Work out the finished part from the listing and answer in its coordinate system (mm). Face numbers are marked on the shaded views. Coordinates: 2 decimals unless noted, no trailing zeros. Write each loop counter-clockwise with the first axis right and the second up, starting at its lowest first coordinate (ties: lowest second). Pieces come first, ordered by that corner, then holes. Notation, with made-up numbers: (57.5, 46.5) - (66.5, 46.5) arc R11 ccw to (66.5, 56.5) - close; hole circle Ø2 at (77, -37.5). An arc over 180 degrees is marked (long way). Use one line per item in the form item = value. Start each with the question number.
Item 1: A cutting plane is placed at B-B (z = -4). Write down the section's boundary in (x, y).
Item 2: A cutting plane is placed at C-C (x = -4). Write down the section's boundary in (y, z).
Item 3: A cutting plane is placed at A-A (y = 1.5). Give the number of separate pieces and of enclosed holes in the cut face, then the cut area to 3 significant figures.
Item 4: Determine the mould class of the marked faces 1 and 2 for opening direction X: released by +X, released by -X, zero draft, split by the parting line, or undercut.
Item 5: A cutting plane is placed at D-D (x = -103.5). Write down the section's boundary in (y, z), then the cut area to 3 significant figures.
Item 6: Consider probe 1 along X at (y, z) = (1.9, -4); probe 2 along X at (y, z) = (-0.4, -35.9); probe 3 along Z at (x, y) = (-4, -0.4). Determine where each line is inside the solid, lowest interval first.
Item 7: Given pin 1 (4 mm diameter, centred on x = -99, z = -10, fed in from -Y), flat-ended and moving along its own axis, determine where the tip first touches the part or whether it passes through.
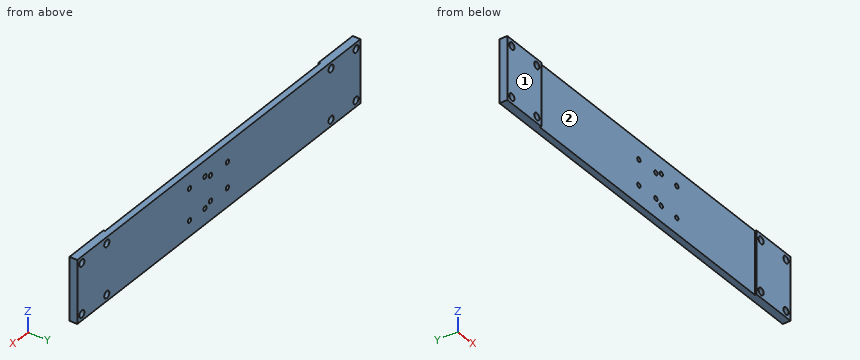
from build123d import *
from build123d.topology import SkipClean

# Parameters (mm, degrees)
SKETCH_1_W          = 250
SKETCH_1_H          = 39.9
EXTRUDE_1_DEPTH     = 4
SKETCH_2_R          = 1.45
CUT_EXTRUDE_1_DEPTH = 12
SKETCH_3_R          = 1.45
CUT_EXTRUDE_2_DEPTH = 12
SKETCH_7_R          = 2.25
CUT_EXTRUDE_6_DEPTH = 20
SKETCH_8_W          = 30
SKETCH_8_H          = 39.9
SKETCH_8_R          = 2.25
EXTRUDE_2_DEPTH     = 1


with BuildPart() as part:
    # Sketch 1 → Extrude 1 (new body)
    with BuildSketch(Plane(origin=(0, 0, 0), x_dir=(1, 0, 0), z_dir=(0, 1, 0))):
        with Locations((-125, 19.95)):
            Rectangle(SKETCH_1_W, SKETCH_1_H)
    extrude(amount=EXTRUDE_1_DEPTH)

    # Sketch 2 → Cut-Extrude 1 (cut)
    with BuildSketch(Plane(origin=(0, 4, 0), x_dir=(1, 0, 0), z_dir=(0, 1, 0))):
        with Locations(Location((-132.5, 27.95, 0), (0, 0, 270))):
            Circle(SKETCH_2_R)
        with Locations(Location((-117.5, 27.95, 0), (0, 0, 270))):
            Circle(SKETCH_2_R)
        with Locations(Location((-117.5, 11.95, 0), (0, 0, 270))):
            Circle(SKETCH_2_R)
        with Locations(Location((-132.5, 11.95, 0), (0, 0, 270))):
            Circle(SKETCH_2_R)
    extrude(amount=-CUT_EXTRUDE_1_DEPTH, mode=Mode.SUBTRACT)

    # Sketch 3 → Cut-Extrude 2 (cut)
    with BuildSketch(Plane(origin=(-275.091791604, 0, 105.376222054), x_dir=(-0.9999983055135633, 0, 0.0018409155336922224), z_dir=(0, -1, 0))):
        with Locations(Location((-162.553914397, 115.077169025, 0), (0, 0, 90.10547675))):
            Circle(SKETCH_3_R)
        with Locations(Location((-162.590548616, 134.977135305, 0), (0, 0, 90.10547675))):
            Circle(SKETCH_3_R)
        with Locations(Location((-176.303891098, 115.051856436, 0), (0, 0, 90.10547675))):
            Circle(SKETCH_3_R)
        with Locations(Location((-176.340525317, 134.951822716, 0), (0, 0, 90.10547675))):
            Circle(SKETCH_3_R)
    extrude(amount=-CUT_EXTRUDE_2_DEPTH, mode=Mode.SUBTRACT)

    # Sketch 7 → Cut-Extrude 6 (cut)
    with BuildSketch(Plane(origin=(0, 4, 0), x_dir=(1, 0, 0), z_dir=(0, 1, 0))):
        with Locations(Location((-246, 35.9, 0), (0, 0, 270))):
            Circle(SKETCH_7_R)
        with Locations(Location((-224, 35.9, 0), (0, 0, 270))):
            Circle(SKETCH_7_R)
        with Locations(Location((-224, 4, 0), (0, 0, 270))):
            Circle(SKETCH_7_R)
        with Locations(Location((-246, 4, 0), (0, 0, 270))):
            Circle(SKETCH_7_R)
        with Locations(Location((-4, 4, 0), (0, 0, 270))):
            Circle(SKETCH_7_R)
        with Locations(Location((-26, 4, 0), (0, 0, 270))):
            Circle(SKETCH_7_R)
        with Locations(Location((-26, 35.9, 0), (0, 0, 270))):
            Circle(SKETCH_7_R)
        with Locations(Location((-4, 35.9, 0), (0, 0, 270))):
            Circle(SKETCH_7_R)
    extrude(amount=-CUT_EXTRUDE_6_DEPTH, mode=Mode.SUBTRACT)

    # Sketch 8 → Extrude 2 (add)
    # profile 1 of 2: a face of its own
    with SkipClean():  # the faces are left unmerged after this step: merging them gives an invalid solid
        with BuildSketch(Plane.XZ):
            with Locations((-235, -19.95)):
                Rectangle(SKETCH_8_W, SKETCH_8_H)
            with Locations(Location((-224, -35.9, 0), (0, 0, 90))):
                Circle(SKETCH_8_R, mode=Mode.SUBTRACT)
            with Locations(Location((-246, -35.9, 0), (0, 0, 90))):
                Circle(SKETCH_8_R, mode=Mode.SUBTRACT)
            with Locations(Location((-224, -4, 0), (0, 0, 270))):
                Circle(SKETCH_8_R, mode=Mode.SUBTRACT)
            with Locations(Location((-246, -4, 0), (0, 0, 270))):
                Circle(SKETCH_8_R, mode=Mode.SUBTRACT)
        # profile 2 of 2: a face of its own
        with BuildSketch(Plane.XZ):
            with Locations((-15, -19.95)):
                Rectangle(SKETCH_8_W, SKETCH_8_H)
            with Locations(Location((-4, -35.9, 0), (0, 0, 270))):
                Circle(SKETCH_8_R, mode=Mode.SUBTRACT)
            with Locations(Location((-26, -35.9, 0), (0, 0, 270))):
                Circle(SKETCH_8_R, mode=Mode.SUBTRACT)
            with Locations(Location((-4, -4, 0), (0, 0, 90))):
                Circle(SKETCH_8_R, mode=Mode.SUBTRACT)
            with Locations(Location((-26, -4, 0), (0, 0, 90))):
                Circle(SKETCH_8_R, mode=Mode.SUBTRACT)
        extrude(amount=EXTRUDE_2_DEPTH)
    add(part.part.scale(1), mode=Mode.REPLACE)  # the faces are merged on a copy


solid = part.part
Answer:
q1.outline = (-250, -1) - (-248.25, -1) - (-248.25, 4) - (-250, 4) - close; (-243.75, -1) - (-226.25, -1) - (-226.25, 4) - (-243.75, 4) - close; (-221.75, -1) - (-220, -1) - (-220, 0) - (-30, 0) - (-30, -1) - (-28.25, -1) - (-28.25, 4) - (-221.75, 4) - close; (-23.75, -1) - (-6.25, -1) - (-6.25, 4) - (-23.75, 4) - close; (-1.75, -1) - (0, -1) - (0, 4) - (-1.75, 4) - close
q2.outline = (-1, -39.9) - (4, -39.9) - (4, -38.15) - (-1, -38.15) - close; (-1, -33.65) - (4, -33.65) - (4, -6.25) - (-1, -6.25) - close; (-1, -1.75) - (4, -1.75) - (4, 0) - (-1, 0) - close
q3.separate_pieces = 1
q3.enclosed_holes = 16
q3.area = 9,790 mm²
q4.face_1 = zero draft
q4.face_2 = undercut
q5.outline = (0, -39.9) - (4, -39.9) - (4, 0) - (0, 0) - close
q5.area = 160 mm²
q6.probe_1 = -250 to -248.25, -243.75 to -226.25, -221.75 to -28.25, -23.75 to -6.25, -1.75 to 0
q6.probe_2 = -250 to -248.25, -243.75 to -226.25, -221.75 to -220, -30 to -28.25, -23.75 to -6.25, -1.75 to 0
q6.probe_3 = -39.9 to -38.15, -33.65 to -6.25, -1.75 to 0
q7.pin_1 = 0
